Verification items for the finished model (mm, model axes). A direction names the side the tool comes from. Coordinates: 2 decimals unless noted, no trailing zeros. Order: outer loops, then holes, each group sorted by start corner. A loop starts at its lowest first (then second) coordinate and runs counter-clockwise, first axis right, second up. Notation, with made-up numbers: M 4,85.25 L 45,85.25 A7 cw 45,97.25 Z; hole C -15,-38 d11. An arc over 180 degrees is marked long. Write item = value, one per line.
```python
from build123d import *

# Parameters (mm, degrees)
CROQUIS1_R              = 1.7
SALIENTE_EXTRUIR1_DEPTH = 5
CROQUIS3_R              = 2.95
CORTAR_EXTRUIR1_DEPTH   = 3
SKETCH1_W               = 3
SKETCH1_H               = 9
BOSS_EXTRUDE1_DEPTH     = 9
CUT_EXTRUDE3_DEPTH      = 10
CUT_EXTRUDE3_DEPTH_BACK = 73
SKETCH2_R               = 1.7
SKETCH4_R               = 2.95
CUT_EXTRUDE4_DEPTH      = 1
CUT_EXTRUDE5_START      = -1
SKETCH5_R               = 2.95
CUT_EXTRUDE5_DEPTH      = 1


with BuildPart() as part:
    # Croquis1 → Saliente-Extruir1 (new body)
    with BuildSketch(Plane(origin=(0, 0, 0), x_dir=(1, 0, 0), z_dir=(0, 1, 0))):
        with BuildLine():
            Line((-31.859064644, -3), (-27.335873866, -3))
            ThreePointArc((-27.335873866, -3), (-27.45893781, -1.502243105), (-27.5, 0))
            Line((-27.5, 0), (-21, 0))
            ThreePointArc((-21, 0), (-20.697569753, 3.551141553), (-19.798989873, 7))
            Line((-19.798989873, 7), (-26.594172294, 7))
            ThreePointArc((-26.594172294, 7), (0, 27.5), (26.594172294, 7))
            Line((26.594172294, 7), (19.798989873, 7))
            ThreePointArc((19.798989873, 7), (20.697569753, 3.551141553), (21, 0))
            Line((21, 0), (27.5, 0))
            ThreePointArc((27.5, 0), (27.45893781, -1.502243105), (27.335873866, -3))
            Line((27.335873866, -3), (31.859064644, -3))
            ThreePointArc((31.859064644, -3), (0, 32), (-31.859064644, -3))
        make_face()
        with Locations(Location((-25, 3.5, 0), (0, 0, 270))):
            Circle(CROQUIS1_R, mode=Mode.SUBTRACT)
        with Locations(Location((25, 3.5, 0), (0, 0, 270))):
            Circle(CROQUIS1_R, mode=Mode.SUBTRACT)
    extrude(amount=SALIENTE_EXTRUIR1_DEPTH)

    # Croquis3 → Cortar-Extruir1 (cut)
    with BuildSketch(Plane(origin=(0, 5, 0), x_dir=(1, 0, 0), z_dir=(0, 1, 0))):
        with Locations(Location((-25, 3.5, 0), (0, 0, 270))):
            Circle(CROQUIS3_R)
        with Locations(Location((25, 3.5, 0), (0, 0, 270))):
            Circle(CROQUIS3_R)
    extrude(amount=-CORTAR_EXTRUIR1_DEPTH, mode=Mode.SUBTRACT)

    # Sketch1 → Boss-Extrude1 (add)
    with BuildSketch(Plane(origin=(0, 5, 0), x_dir=(1, 0, 0), z_dir=(0, 1, 0))):
        with Locations((-29.5, 2)):
            Rectangle(SKETCH1_W, SKETCH1_H)
        with Locations((29.5, 2)):
            Rectangle(SKETCH1_W, SKETCH1_H)
    extrude(amount=BOSS_EXTRUDE1_DEPTH)

    # Sketch2 → Cut-Extrude3 (cut, two sides: drawn at the far end of the back side and taken through both)
    with BuildSketch(Plane.ZY.offset(31).offset(-CUT_EXTRUDE3_DEPTH_BACK)):
        with Locations(Location((-2, 9.5, 0), (0, 0, 180))):
            Circle(SKETCH2_R)
    extrude(amount=CUT_EXTRUDE3_DEPTH + CUT_EXTRUDE3_DEPTH_BACK, mode=Mode.SUBTRACT)

    # Sketch4 → Cut-Extrude4 (cut)
    with BuildSketch(Plane.ZY.offset(31)):
        with Locations((-2, 9.5)):
            Circle(SKETCH4_R)
    extrude(amount=-CUT_EXTRUDE4_DEPTH, mode=Mode.SUBTRACT)

    # Sketch5 → Cut-Extrude5 (cut)
    with BuildSketch(Plane(origin=(31, 0, 0), x_dir=(0, 0, -1), z_dir=(1, 0, 0)).offset(CUT_EXTRUDE5_START)):
        with Locations(Location((2, 9.5, 0), (0, 0, 180))):
            Circle(SKETCH5_R)
    extrude(amount=CUT_EXTRUDE5_DEPTH, mode=Mode.SUBTRACT)


solid = part.part
```
Item 1: Sectioned sample at A-A, the plane y = 9.5. Enter the section's corners in (x, z).
Report:
outline = M -31,-6.5 L -28,-6.5 L -28,-3.7 L -30,-3.7 L -30,-4.95 L -31,-4.95 Z; M -31,0.95 L -30,0.95 L -30,-0.3 L -28,-0.3 L -28,2.5 L -31,2.5 Z; M 28,-6.5 L 31,-6.5 L 31,-4.95 L 30,-4.95 L 30,-3.7 L 28,-3.7 Z; M 28,-0.3 L 30,-0.3 L 30,0.95 L 31,0.95 L 31,2.5 L 28,2.5 Z
Item 2: Release check for a two-part mould opening along Y. For faces 1 (the flat face through (29, 14, -2)), 2 (the flat face through (-30, 7.6, -2)), 3 (the flat face through (-30, 9, 2.5)) record: pulls with the +Y half, pulls with the -Y half, needs draft (parallel to the pull), parting line crosses it, or undercut.
Report:
face_1 = pulls with the +Y half
face_2 = undercut
face_3 = needs draft
Item 3: Sectioned sample at D-D, the plane z = -21.5. Enter the section's corners in (x, y).
Report:
outline = M -23.7,0 L -17.15,0 L -17.15,5 L -23.7,5 Z; M 17.15,0 L 23.7,0 L 23.7,5 L 17.15,5 Z
Item 4: Sectioned sample at B-B, the plane z = -14. Enter the section's corners in (x, y).
Report:
outline = M -28.77,0 L -23.67,0 L -23.67,5 L -28.77,5 Z; M 23.67,0 L 28.77,0 L 28.77,5 L 23.67,5 Z
Item 5: Gauge pin test, flat ends, axial feed: pin 1 (0.9 mm diameter, centred on x = 30, y = 11.5, fed in from -Z); pin 2 (0.9 mm diameter, centred on x = -29, y = 9, fed in from +Z); pin 3 (3 mm diameter, centred on y = 8.5, z = -2, fed in from -X); pin 4 (5 mm diameter, centred on x = -19.5, z = -23.5, fed in from -Y). Record the tip position at first contact, or that the pin passes through.
Report:
pin_1 = -6.5
pin_2 = 2.5
pin_3 = -30
pin_4 = 0
Item 6: Sectioned sample at C-C, the plane y = 1. Enter the section's corners in (x, z).
Report:
outline = M -31.86,3 A32 ccw long 31.86,3 L 27.34,3 A27.5 cw 27.5,0 L 21,0 A21 cw 19.8,-7 L 26.59,-7 A27.5 cw -26.59,-7 L -19.8,-7 A21 cw -21,0 L -27.5,0 A27.5 cw -27.34,3 Z; hole C -25,-3.5 d3.4; hole C 25,-3.5 d3.4
Item 7: Scan lines: L1, parallel to X at y = 3.25, z = -4.5; L2, parallel to X at y = 2.75, z = 0.5; L3, parallel to X at y = 7, z = -4. Record each from-to range of solid material in increasing order. Write a range as from..to.
Report:
L1 = -31.68..-27.78, -22.22..-20.51, 20.51..22.22, 27.78..31.68
L2 = -32..-27.5, 27.5..32
L3 = -31..-28, 28..31
Item 8: Tool access check on faces 4 (the flat face through (29, 9, 2.5)), 5 (the flat face through (23, 2, -4)), 6 (the cylindrical face through (-27.458, 2.465, 1.523)). Record the directions out of +Z, -Z, +X, -X, +Y, -Y that give a thin tool (end or side, any length) a straight path to the whole face; none if there is none.
Report:
face_4 = +Z, +X, -X, +Y
face_5 = +Y
face_6 = +Y, -Y
